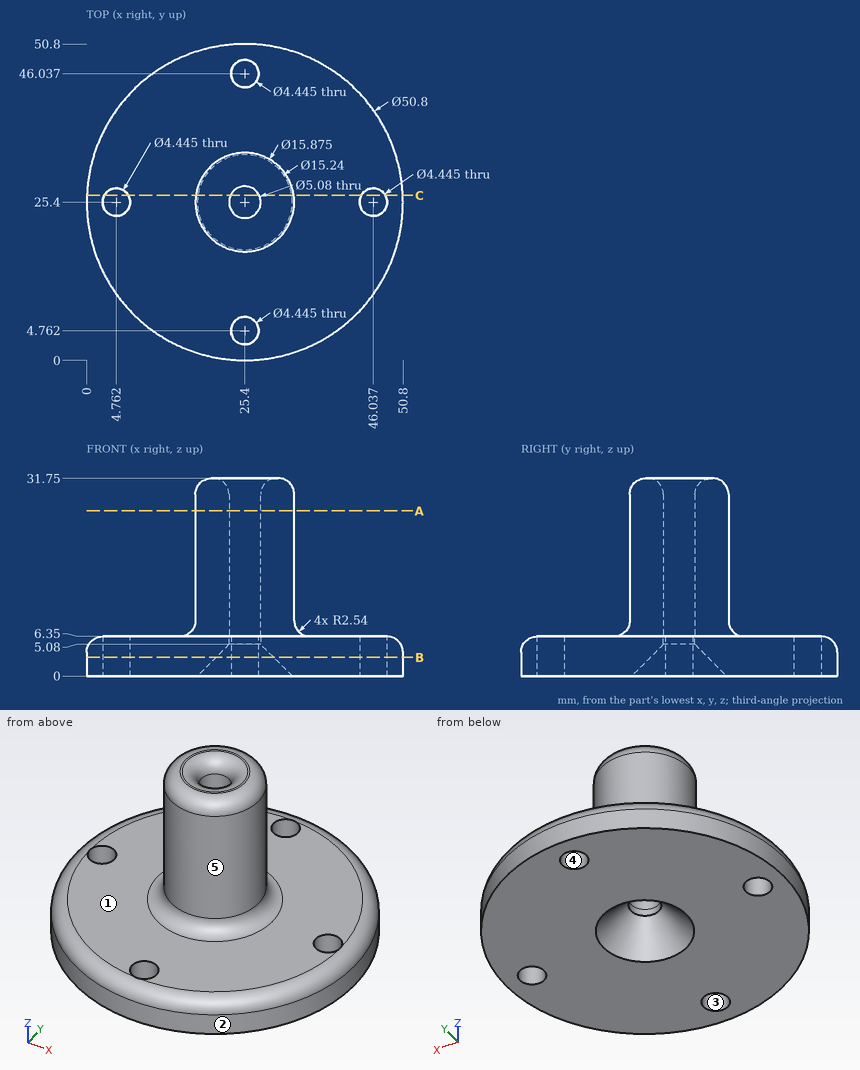
Could you check a few things on this drawing? It's one solid part, dimensions in mm from its lowest x, y, z. A direction names the side the tool comes from. Coordinates: 2 decimals unless noted, no trailing zeros. Order: outer loops, then holes, each group sorted by start corner. A loop starts at its lowest first (then second) coordinate and runs counter-clockwise, first axis right, second up. Notation, with made-up numbers: (85.5, 33.25) - (112.5, 33.25) arc R23 cw to (112.5, 42.25) - close; hole circle Ø6 at (-24, 65). An arc over 180 degrees is marked (long way). Answer as a JSON object with one key per item and string values. Group by question number.
Q1. On a 3-axis mill with a long thin cutter (end or side, diameter ignored), from which of +Z, -Z, +X, -X, +Y, -Y can I reach the whole of each face in a straight line? I mean the marked faces 4 and 5. Say none if no direction works.
Q2. Imagine slicing it at C-C (y = 26.5). Give the number of separate pieces and of enclosed holes in the cut face.
Q3. We'd pull the mould along Y, two halves only. Please class the marked faces 1, 2 and 3: +Y half, -Y half, draft (parallel to the pull), parting line (faces both ways), or undercut.
Q4. I need wall thicknesses on line 1 (Y direction, x = 23.5, z = 2) (1 decimal); line 2 (Y direction, x = 25.4, z = 1.5) (1 decimal); line 3 (Z direction, x = 35, y = 31). Which ranges of each line are inside material? Lowest first, please. Write a range as from..to.
Q5. Imagine slicing it at B-B (z = 3). Please give me the cut outline in (x, y) (1 decimal).
Q6. Will these pins go through, and if not, where does the flat tip stop? P1, Ø5, axis at x = 15, y = 40.5, coming from the +Z side; P2, Ø4, axis at x = 30.5, z = 3.5, coming from the +Y side; P3, Ø6, axis at y = 16.5, z = 9.5, coming from the -X side.
Q7. Imagine slicing it at A-A (z = 26.5). Please give me the cut outline in (x, y) (1 decimal).
Determined:
{
 "1": {"face 4": "+Z, -Z", "face 5": "+Z"},
 "2": {"separate pieces": "4", "enclosed holes": "0"},
 "3": {"face 1": "draft", "face 2": "parting line", "face 3": "undercut"},
 "4": {"line 1": "y = 0.1..3.6, 5.9..20.1, 30.7..44.9, 47.2..50.7", "line 2": "y = 0..2.5, 7..19.3, 31.5..43.8, 48.3..50.8", "line 3": "z = 0..6.35"},
 "5": {"outline": "circle Ø50.8 at (25.4, 25.4); hole circle Ø4.4 at (4.8, 25.4); hole circle Ø9.2 at (25.4, 25.4); hole circle Ø4.4 at (25.4, 4.8); hole circle Ø4.4 at (25.4, 46); hole circle Ø4.4 at (46, 25.4)"},
 "6": {"P1": "stops at z = 6.35", "P2": "stops at y = 50.61", "P3": "stops at x = 20.09"},
 "7": {"outline": "circle Ø15.9 at (25.4, 25.4); hole circle Ø5.1 at (25.4, 25.4)"}
}
